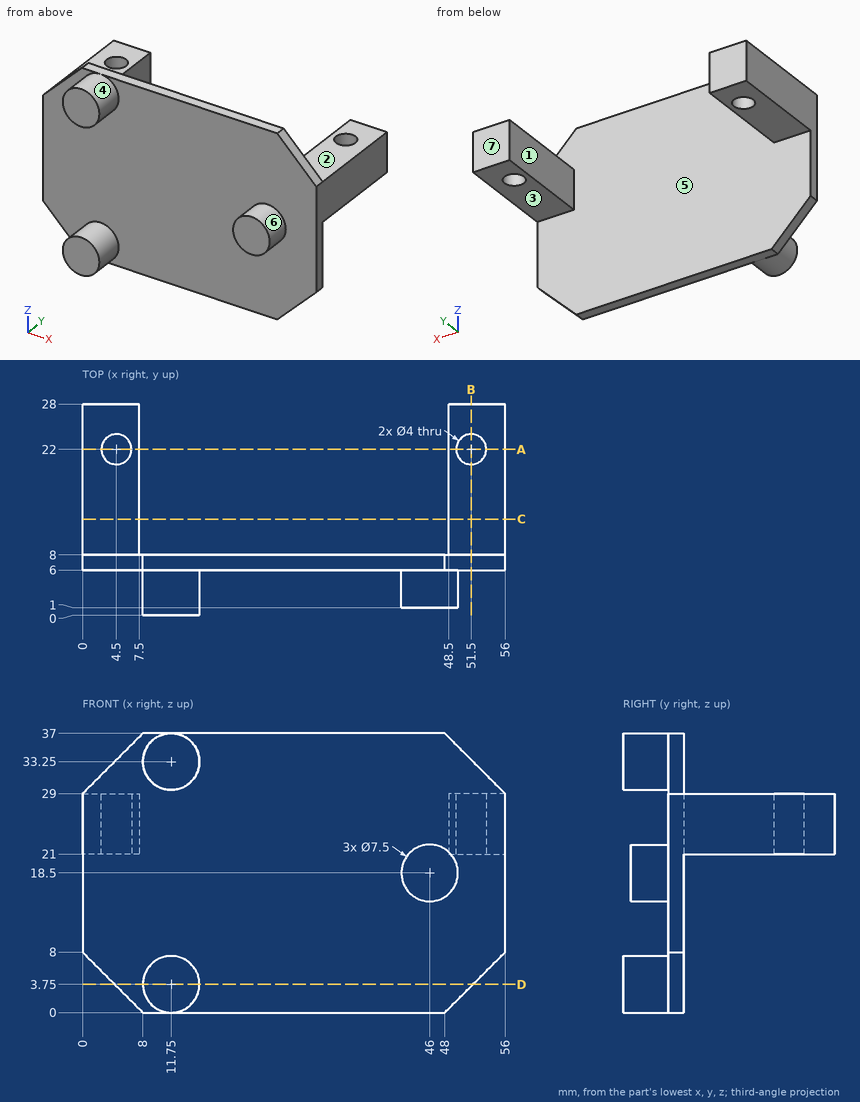
Geometry: see drawing. Coordinates: mm, zero at the bounding-box minimum. A direction names the side the tool comes from. Round coordinates to 2 decimals unless told otherwise and drop trailing zeros. Order: outer loops, then holes, each group sorted by start corner. A loop starts at its lowest first (then second) coordinate and runs counter-clockwise, first axis right, second up. Notation, with made-up numbers: (-15, -38.5) -> (15, -38.5) arc R20 ccw to (15, -11.5) -> close; hole circle Ø2 at (85.5, -36). An arc over 180 degrees is marked (long way). Answer as CSV lines item,"result".
Item 1: Line query: L1, parallel to Y at x = 4.5, z = 23.25; L2, parallel to X at y = 8.75, z = 22; L3, parallel to Y at x = 37, z = 18.5. Output: solid intervals per line, ascending.
A:
L1,"6 to 20, 24 to 28"
L2,"0 to 7.5, 48.5 to 56"
L3,"6 to 8"
Item 2: Reachability of the marked faces 1, 2, 3 and 4 from +Z, -Z, +X, -X, +Y, -Y: full face, straight path, thin tool, end or side. Return the list, or none.
A:
face 1,"+Z, -Z, +Y"
face 2,"+Z, +X, -X, +Y"
face 3,"-Z, +X, -X, +Y"
face 4,"-Y"
Item 3: Section C-C, the plane y = 12.75. Return loops of the section in (x, z), plus the area to 3 significant figures.
A:
outline,"(0, 21) -> (7.5, 21) -> (7.5, 29) -> (0, 29) -> close; (48.5, 21) -> (56, 21) -> (56, 29) -> (48.5, 29) -> close"
area,"120 mm²"
Item 4: Pin query (flat end, axial travel): pin 1 Ø6 at (x, y) = (5.5, 22) entering from +Z; pin 2 Ø2.5 at (x, y) = (4.5, 22) entering from -Z; pin 3 Ø10 at (y, z) = (25, 24) entering from -X; pin 4 Ø4 at (x, z) = (47.5, 18.5) entering from -Y. Return the tip coordinate at first contact, or that it passes through.
A:
pin 1,"z = 29"
pin 2,"through"
pin 3,"x = 0"
pin 4,"y = 1"
Item 5: Section D-D, the plane z = 3.75. Return loops of the section in (x, y), plus the area to 3 significant figures.
A:
outline,"(4.25, 6) -> (8, 6) -> (8, 0) -> (15.5, 0) -> (15.5, 6) -> (51.75, 6) -> (51.75, 8) -> (4.25, 8) -> close"
area,"140 mm²"
Item 6: Section A-A, the plane y = 22. Return loops of the section in (x, z).
A:
outline,"(0, 21) -> (2.5, 21) -> (2.5, 29) -> (0, 29) -> close; (6.5, 21) -> (7.5, 21) -> (7.5, 29) -> (6.5, 29) -> close; (48.5, 21) -> (49.5, 21) -> (49.5, 29) -> (48.5, 29) -> close; (53.5, 21) -> (56, 21) -> (56, 29) -> (53.5, 29) -> close"
Item 7: Pull-direction query (X, two-part tool) for the marked faces 5, 6 and 7; classes: pulls with the +X half, pulls with the -X half, needs draft (parallel to the pull), parting line crosses it, or undercut.
A:
face 5,"undercut"
face 6,"parting line crosses it"
face 7,"needs draft"
Item 8: Section B-B, the plane x = 51.5. Return loops of the section in (y, z), plus the area to 3 significant figures.
A:
outline,"(6, 3.5) -> (8, 3.5) -> (8, 21) -> (20, 21) -> (20, 29) -> (8, 29) -> (8, 33.5) -> (6, 33.5) -> close; (24, 21) -> (28, 21) -> (28, 29) -> (24, 29) -> close"
area,"188 mm²"
